Part model, mm, in its own coordinate system. Face numbers are marked on the shaded views. A direction names the side the tool comes from. Round coordinates to 2 decimals unless told otherwise and drop trailing zeros. Write each loop counter-clockwise with the first axis right and the second up, starting at its lowest first coordinate (ties: lowest second). Pieces come first, ordered by that corner, then holes.
Autodesk Inventor part; units mm, degrees
ref_plane "YZ Plane" through (0, 0, 0) normal (1, 0, 0) x (0, 1, 0)
ref_plane "XZ Plane" through (0, 0, 0) normal (0, 1, 0) x (-1, 0, 0)
ref_plane "XY Plane" through (0, 0, 0) normal (0, 0, 1) x (1, 0, 0)
sketch "Sketch1" plane through (0, 0, 0) normal (0, 1, 0) x (-1, 0, 0)
  line L0 (0, 0) -> (0, -11.938)
  line L1 (-15.24, 3.3655) -> (-15.24, -15.3035)
  line L2 (0, 0) -> (-15.24, 3.3655)
  line L3 (0, -11.938) -> (-15.24, -15.3035)
  line L4 (-15.24, 3.3655) -> (-19.05, 3.3655)
  line L5 (-19.05, 3.3655) -> (-19.05, 2.0955)
  line L6 (-19.05, 2.0955) -> (-15.24, 2.0955)
  line L7 (-15.24, 2.0955) -> (-15.24, 3.3655)
  line L8 (-15.24, -15.3035) -> (-19.05, -15.3035)
  line L9 (-19.05, -15.3035) -> (-19.05, -14.0335)
  line L10 (-19.05, -14.0335) -> (-15.24, -14.0335)
  line L11 (-15.24, -14.0335) -> (-15.24, -15.3035)
  line L12 (0, 0) -> (0, 3.175)
  line L13 (-15.24, 3.3655) -> (-15.24, 6.5405)
  line L14 (0, -11.938) -> (0, -15.113)
  line L15 (-15.24, -15.3035) -> (-15.24, -18.4785)
  line L16 (-15.24, -18.4785) -> (0, -15.113)
  line L17 (0, 3.175) -> (-15.24, 6.5405)
  line L18 (-15.24, 6.5405) -> (-34.29, 6.5405)
  line L19 (-19.05, 3.3655) -> (-34.29, 3.3655)
  line L20 (-34.29, 3.3655) -> (-34.29, 6.5405)
  line L21 (-15.24, -18.4785) -> (-34.29, -18.4785)
  line L22 (-34.29, -18.4785) -> (-34.29, -15.3035)
  line L23 (-34.29, -15.3035) -> (-19.05, -15.3035)
  line L24 (-34.29, 6.5405) -> (-37.465, 6.5405)
  line L25 (-37.465, 6.5405) -> (-37.465, -18.4785)
  line L26 (-37.465, -18.4785) -> (-34.29, -18.4785)
  line L27 (-34.29, -18.4785) -> (-34.29, 6.5405)
  dimension "d0" = 11.938
  dimension "d1" = 15.24
  dimension "d2" = 18.669
  dimension "d3" = 3.3655
  dimension "d4" = 3.81
  dimension "d5" = 1.27
  dimension "d6" = 3.81
  dimension "d7" = 1.27
  dimension "d8" = 3.175
  dimension "d9" = 3.175
  dimension "d10" = 3.175
  dimension "d11" = 3.175
  dimension "d12" = 19.05
  dimension "d13" = 3.175
extrude "Extrusion1" add sketch "Sketch1" along normal blind 6.985 contours L2 L13 L17 L12 | L14 L16 L15 L3 | L1 L6 L5 L4 | L4 L19 L20 L18 L13 | L8 L9 L10 L1 | L15 L21 L22 L23 L8 | L27 L22 L26 L25 L24 L20
sketch "Sketch2" plane through (0, 6.985, 0) normal (0, 1, 0) x (1, 0, 0)
  line L0 (0, 11.938) -> (15.24, 15.3035)
  line L1 (15.24, 15.3035) -> (15.24, 14.0335)
  line L2 (15.24, 14.0335) -> (19.05, 14.0335)
  line L3 (19.05, 14.0335) -> (19.05, 15.3035)
  line L4 (19.05, 15.3035) -> (34.29, 15.3035)
  line L5 (34.29, 15.3035) -> (34.29, -3.3655)
  line L6 (34.29, -3.3655) -> (19.05, -3.3655)
  line L7 (19.05, -3.3655) -> (19.05, -2.0955)
  line L8 (19.05, -2.0955) -> (15.24, -2.0955)
  line L9 (15.24, -2.0955) -> (15.24, -3.3655)
  line L10 (15.24, -3.3655) -> (0, 0)
  line L11 (0, 0) -> (0, -3.175)
  line L12 (0, -3.175) -> (15.24, -6.5405)
  line L13 (15.24, -6.5405) -> (37.465, -6.5405)
  line L14 (37.465, -6.5405) -> (37.465, 18.4785)
  line L15 (37.465, 18.4785) -> (15.24, 18.4785)
  line L16 (15.24, 18.4785) -> (0, 15.113)
  line L17 (0, 15.113) -> (0, 11.938)
  line L18 (0, 0) -> (0, -3.175)
  line L19 (15.24, 18.4785) -> (0, 15.113)
  line L20 (0, -3.175) -> (0, 15.113)
extrude "Extrusion2" add sketch "Sketch2" along normal blind 1.5875
sketch "Sketch3" plane through (37.465, 0, 6.5405) normal (1, 0, 0) x (0, 0, -1)
  line L0 (21.844, 0) -> (21.844, 6.985)
  line L1 (21.844, 0) -> (3.175, 0)
  line L2 (3.175, 0) -> (3.175, 6.985)
  line L3 (21.844, 6.985) -> (3.175, 6.985)
  line L4 (3.175, 0) -> (3.175, 6.985)
  line L5 (3.175, 4.445) -> (9.525, 4.445)
  line L6 (9.525, 4.445) -> (9.525, 0)
  line L7 (9.525, 0) -> (3.175, 0)
  line L8 (3.175, 0) -> (3.175, 4.445)
  line L9 (21.844, 0) -> (21.844, 6.985)
  line L10 (21.844, 0) -> (15.494, 0)
  line L11 (15.494, 0) -> (15.494, 4.445)
  line L12 (15.494, 4.445) -> (21.844, 4.445)
  line L13 (21.844, 4.445) -> (21.844, 0)
  line L14 (0, 0) -> (25.019, 0)
  point P0 (6.5405, 0)
  dimension "d18" = 6.35
  dimension "d19" = 6.35
  dimension "d20" = 4.445
  dimension "d21" = 4.445
extrude "Extrusion3" cut sketch "Sketch3" against normal blind 3.175 contours L1 L11 L12 L0 | L1 L2 L5 L6
sketch "Sketch5" plane through (0, 6.985, 0) normal (0, -1, 0) x (1, 0, 0)
  circle A0 centre (8.636, -5.969) radius 1.5875
  line L0 (0, 0) -> (0, 3.175)
  line L1 (0, -11.938) -> (0, 0)
  dimension "d24" = 3.175
  dimension "d25" = 8.636
extrude "Extrusion4" cut sketch "Sketch5" against normal blind 25.4
sketch "Sketch6" plane through (0, 8.5725, 0) normal (0, 1, 0) x (1, 0, 0)
  line L0 (37.465, 18.4785) -> (15.24, 18.4785)
  line L1 (15.24, -6.5405) -> (37.465, -6.5405)
  line L2 (15.24, 18.4785) -> (0, 15.113)
  line L3 (15.24, 18.4785) -> (22.86, 18.4785)
  line L4 (22.86, 18.4785) -> (22.86, 26.0985)
  line L5 (22.86, 26.0985) -> (15.24, 26.0985)
  line L6 (15.24, 26.0985) -> (15.24, 18.4785)
  line L7 (15.24, -6.5405) -> (22.86, -6.5405)
  line L8 (22.86, -6.5405) -> (22.86, -14.1605)
  line L9 (22.86, -14.1605) -> (15.24, -14.1605)
  line L10 (15.24, -14.1605) -> (15.24, -6.5405)
  point P0 (0, 0)
  dimension "d28" = 7.62
  dimension "d29" = 7.62
  dimension "d30" = 7.62
  dimension "d31" = 7.62
extrude "Extrusion5" add sketch "Sketch6" against normal blind 3.175
sketch "Sketch7" plane through (0, 5.3975, 0) normal (0, -1, 0) x (1, 0, 0)
  line L0 (22.86, 6.5405) -> (15.24, 6.5405)
  line L1 (22.86, 6.5405) -> (22.86, 14.1605)
  line L2 (22.86, 14.1605) -> (15.24, 14.1605)
  line L3 (15.24, 14.1605) -> (15.24, 6.5405)
  line L4 (15.24, -18.4785) -> (22.86, -18.4785)
  line L5 (15.24, -18.4785) -> (15.24, -26.0985)
  line L6 (15.24, -26.0985) -> (22.86, -26.0985)
  line L7 (22.86, -26.0985) -> (22.86, -18.4785)
  circle A0 centre (19.05, 10.3505) radius 1.5875
  circle A1 centre (19.05, -22.2885) radius 1.5875
  point P0 (0, 0)
  dimension "d34" = 3.175
  dimension "d35" = 3.175
extrude "Extrusion6" cut sketch "Sketch7" against normal through all contours A0 | A1
chamfer "Chamfer1" distance 1.27 angle 45 2 edges at (17.4625, 5.3975, 10.3505) (17.4625, 5.3975, -22.2885)
fillet "Fillet1" radius 3.175 8 edges at (15.24, 6.985, -26.0985) (22.86, 6.985, -26.0985) (15.24, 6.985, -18.4785) (22.86, 6.985, -18.4785) (15.24, 6.985, 6.5405) (15.24, 6.985, 14.1605) (22.86, 6.985, 14.1605) (22.86, 6.985, 6.5405)
equation "\"d3\" = -0.5 * d0 + 0.5 * d2"
properties part number "phototransistorMount1" material "ABS Plastic"
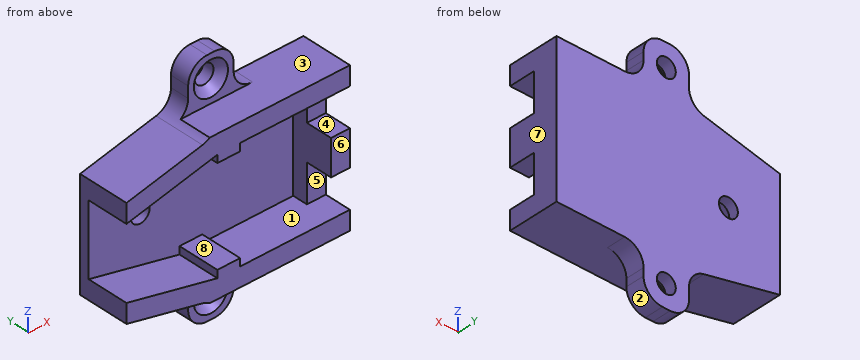
Q1. Tool access for the marked faces 1, 2, 3, 4 and 5: list every direction of +Z, -Z, +X, -X, +Y, -Y with a clear straight run to the whole face (end or side of a thin tool).
Q2. Saw through at B-B, the plane x = 32. Write the cut outline in (y, z) (1 decimal), and give its area (3 significant figures).
Q3. Saw through at A-A, the plane y = 1.25. Give the number of separate pieces and of enclosed holes in the cut face, and give its area (3 significant figures).
Q4. Drop flat-ended pins along their axis: P1, Ø3, axis at x = 4, y = 5, coming from the +Z side; P2, Ø0.6, axis at y = 4.5, z = -14.5, coming from the -X side; P3, Ø3.5, axis at x = 35.5, y = 2.5, coming from the +Z side; P4, Ø5, axis at x = 32, y = 3, coming from the -Z side. Give the stop position or say it passes through.
Q5. Saw through at C-C, the plane x = 8.5. Write the cut outline in (y, z) (1 decimal), and give its area (3 significant figures).
Q6. Two-plate mould, pull along X, no slides. Class the marked faces 6, 7 and 8: released by +X, released by -X, zero draft, split by the parting line, or undercut.
Q7. Wall check: line 1 (Z direction, x = 19.05, y = 7.9); line 2 (Z direction, x = 20.5, y = 2); line 3 (Z direction, x = 36, y = 5). Give the ranges that are in metal, low to high.
Computed:
1. face 1: -Y
1. face 2: -Z, +X, +Y, -Y
1. face 3: +Z, +X, -Y
1. face 4: +X, -X, -Y
1. face 5: +X, -Y
2. outline: (0, -18.5) - (8.6, -18.5) - (8.6, 6.5) - (0, 6.5) - (0, 3.4) - (7, 3.4) - (7, -15.3) - (0, -15.3) - close
2. area: 84.1 mm2
3. separate pieces: 3
3. enclosed holes: 0
3. area: 267 mm2
4. P1: stops at z = 4.39
4. P2: stops at x = 0
4. P3: stops at z = 6.54
4. P4: stops at z = -18.48
5. outline: (0, -17) - (8.6, -17) - (8.6, -7.6) - (7, -7.6) - (7, -13.8) - (0, -13.8) - close; (0, 1.9) - (7, 1.9) - (7, -4.4) - (8.6, -4.4) - (8.6, 5.1) - (0, 5.1) - close
5. area: 74.3 mm2
6. face 6: zero draft
6. face 7: released by +X
6. face 8: undercut
7. line 1: z = -26.1 to -23.88, -20.7 to 8.76, 11.94 to 14.16
7. line 2: z = -18.48 to -15.3, 3.37 to 6.54
7. line 3: z = -18.48 to 6.54
